```python
from build123d import *

# Parameters (mm, degrees)
F0_W     = 200
F0_H     = 200
F1_DEPTH = 70
F2_T     = -2
F3_W     = 2
F3_H     = 196
F4_DEPTH = 68
F5_W     = 54
F5_H     = 186
F6_DEPTH = 2


with BuildPart() as f1:
    # F0 (on Top) → F1 (new body)
    with BuildSketch(Plane.XY):
        Rectangle(F0_W, F0_H)
    extrude(amount=F1_DEPTH)

    # F2
    f2_openings = [f1.faces().sort_by_distance(p)[0] for p in [
        (0, 0, 70),
    ]]
    offset(amount=F2_T, openings=f2_openings)

    # F3 (on face) → F4 (join)
    with BuildSketch(Plane.XY.offset(2)):
        with Locations((-33, 0)):
            Rectangle(F3_W, F3_H)
        with Locations((33, 0)):
            Rectangle(F3_W, F3_H)
    extrude(amount=F4_DEPTH)

    # F5 (on face) → F6 (cut, through all)
    with BuildSketch(Plane.XY.offset(2)):
        Polygon((-73, 93), (-93, 93), (-93, 70.5273523927), (-93, 53), (-93, -93), (-39, -93), (-39, 53), (-39, 93), align=None)
        Rectangle(F5_W, F5_H)
        with Locations((66, 0)):
            Rectangle(F5_W, F5_H)
    extrude(amount=-F6_DEPTH, mode=Mode.SUBTRACT)


solid = f1.part
```
Design review of the part built by this model. Coordinates are the model's own, in mm. A direction names the side the tool comes from. Give positions to 0.01 mm unless a question says otherwise; leave off trailing zeros. Loops run counter-clockwise (first coordinate to the right, second up) from the corner with the lowest first, then second, coordinate; pieces in that order, holes last. Notation, with made-up numbers: (13, 59) -> (50, 59) arc R38 cw to (50, 98) -> close; hole circle Ø10 at (-21, 43). An arc over 180 degrees is marked (long way). One line per item, written item: value.
Q1. We need section B-B on x = -85. Give the boundary of the cut face in (y, z), and give its area (3 significant figures).
Numbers:
outline: (-100, 0) -> (-93, 0) -> (-93, 2) -> (-98, 2) -> (-98, 70) -> (-100, 70) -> close; (93, 0) -> (100, 0) -> (100, 70) -> (98, 70) -> (98, 2) -> (93, 2) -> close
area: 300 mm^2
Q2. We need section A-A on y = -18. Give the boundary of the cut face in (x, z), and give its area (3 significant figures).
Numbers:
outline: (-100, 0) -> (-93, 0) -> (-93, 2) -> (-98, 2) -> (-98, 70) -> (-100, 70) -> close; (-39, 0) -> (-27, 0) -> (-27, 2) -> (-32, 2) -> (-32, 70) -> (-34, 70) -> (-34, 2) -> (-39, 2) -> close; (27, 0) -> (39, 0) -> (39, 2) -> (34, 2) -> (34, 70) -> (32, 70) -> (32, 2) -> (27, 2) -> close; (93, 0) -> (100, 0) -> (100, 70) -> (98, 70) -> (98, 2) -> (93, 2) -> close
area: 620 mm^2
Q3. Machinability: for faces 4 (the flat face through (66, -98, 36)), 5 (the flat face through (100, -1, 35)), which of the approach directions +Z, -Z, +X, -X, +Y, -Y give a long, thin tool a straight path to every point of the face, cutting with its end or side? Answer none if there is none.
Numbers:
face 4: +Z
face 5: +Z, -Z, +X, +Y, -Y
Q4. For L1, parallel to X at y = 66, z = 11; L2, parallel to Y at x = -84, z = 5; L3, parallel to Z at x = 37, y = 72, list the stretches that pass through material, from the lowest coordinate up.
Numbers:
L1: x = -100 to -98, -34 to -32, 32 to 34, 98 to 100
L2: y = -100 to -98, 98 to 100
L3: z = 0 to 2
Q5. We need section C-C on z = 12.5. Give the boundary of the cut face in (x, y), and give its area (3 significant figures).
Numbers:
outline: (-100, -100) -> (100, -100) -> (100, 100) -> (-100, 100) -> close; hole (-98, -98) -> (-34, -98) -> (-34, 98) -> (-98, 98) -> close; hole (-32, -98) -> (32, -98) -> (32, 98) -> (-32, 98) -> close; hole (34, -98) -> (98, -98) -> (98, 98) -> (34, 98) -> close
area: 2,370 mm^2
Q6. Draft analysis for pull direction X (two halves, no side actions). For faces 1 (the flat face through (32, -1, 36)), 2 (the flat face through (-100, -1, 35)), 3 (the flat face through (-1, -100, 35)), state which applies: pulls with the +X half, pulls with the -X half, needs draft (parallel to the pull), parting line crosses it, or undercut.
Numbers:
face 1: undercut
face 2: pulls with the -X half
face 3: needs draft
